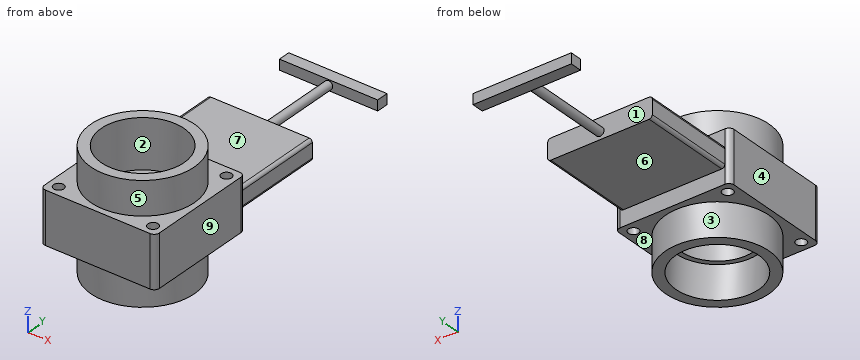
```python
from build123d import *

# Parameters (mm, degrees)
F0_R           = 50.00625
F0_R_2         = 40
F1_DEPTH       = 114.3
F3_R           = 50.00625
F4_DEPTH       = 25
F4_DEPTH_BACK  = 25
F5_R           = 5
F6_DEPTH       = 82.151
F8_DEPTH       = 90
F9_R           = 4
F10_DEPTH      = 85
F11_W          = 95
F11_H          = 10
F11_R          = 4
F12_DEPTH      = 11.51
F13_R          = 40
F13_R_2        = 35
F14_DEPTH      = 10
F14_DEPTH_BACK = 25


with BuildPart() as f1:
    # F0 (on Top) → F1 (new body)
    with BuildSketch(Plane.XY):
        Circle(F0_R)
        Circle(F0_R_2, mode=Mode.SUBTRACT)
    extrude(amount=F1_DEPTH)

    # F3 (on offset) → F4 (join, two sides)
    with BuildSketch(Plane.XY.offset(57.15)) as f4_sk:
        with BuildLine():
            ThreePointArc((55.5625, 50.5625), (54.0980339059, 54.0980339059), (50.5625, 55.5625))
            Line((50.5625, 55.5625), (-50.5625, 55.5625))
            ThreePointArc((-50.5625, 55.5625), (-54.0980339059, 54.0980339059), (-55.5625, 50.5625))
            Line((-55.5625, 50.5625), (-55.5625, -50.5625))
            ThreePointArc((-55.5625, -50.5625), (-54.0980339059, -54.0980339059), (-50.5625, -55.5625))
            Line((-50.5625, -55.5625), (50.5625, -55.5625))
            ThreePointArc((50.5625, -55.5625), (54.0980339059, -54.0980339059), (55.5625, -50.5625))
            Line((55.5625, -50.5625), (55.5625, 50.5625))
        make_face()
        Circle(F3_R, mode=Mode.SUBTRACT)
    extrude(amount=F4_DEPTH)
    extrude(f4_sk.sketch, amount=-F4_DEPTH_BACK)

    # F5 (on face) → F6 (cut, through all)
    with BuildSketch(Plane.XY.offset(82.15)):
        with Locations((-45.5625, 45.5625)):
            Circle(F5_R)
        with Locations((-45.5625, -45.5625)):
            Circle(F5_R)
        with Locations((45.5625, -45.5625)):
            Circle(F5_R)
        with Locations((45.5625, 45.5625)):
            Circle(F5_R)
    extrude(amount=-F6_DEPTH, mode=Mode.SUBTRACT)

    # F7 (on face) → F8 (join)
    with BuildSketch(Plane(origin=(0, 55.5625, 0), x_dir=(-1, 0, 0), z_dir=(0, 1, 0))):
        with BuildLine():
            Line((-47.5625, 47.15), (47.5625, 47.15))
            ThreePointArc((47.5625, 47.15), (49.6838203436, 48.0286796564), (50.5625, 50.15))
            Line((50.5625, 50.15), (50.5625, 64.15))
            ThreePointArc((50.5625, 64.15), (49.6838203436, 66.2713203436), (47.5625, 67.15))
            Line((47.5625, 67.15), (-47.5625, 67.15))
            ThreePointArc((-47.5625, 67.15), (-49.6838203436, 66.2713203436), (-50.5625, 64.15))
            Line((-50.5625, 64.15), (-50.5625, 50.15))
            ThreePointArc((-50.5625, 50.15), (-49.6838203436, 48.0286796564), (-47.5625, 47.15))
        make_face()
    extrude(amount=F8_DEPTH)

    # F9 (on face) → F10 (join)
    with BuildSketch(Plane(origin=(0, 145.5625, 0), x_dir=(-1, 0, 0), z_dir=(0, 1, 0))):
        with Locations((0, 54.15)):
            Circle(F9_R)
    extrude(amount=F10_DEPTH)

    # F11 (on face) → F12 (join)
    with BuildSketch(Plane(origin=(0, 230.5625, 0), x_dir=(-1, 0, 0), z_dir=(0, 1, 0))):
        with Locations((0, 54.15)):
            Rectangle(F11_W, F11_H)
        with Locations((0, 54.15)):
            Circle(F11_R, mode=Mode.SUBTRACT)
        with Locations((0, 54.15)):
            Circle(F11_R)
    extrude(amount=F12_DEPTH)

    # F13 (on offset) → F14 (join, two sides)
    with BuildSketch(Plane.XY.offset(57.15)) as f14_sk:
        Circle(F13_R)
        Circle(F13_R_2, mode=Mode.SUBTRACT)
    extrude(amount=F14_DEPTH)
    extrude(f14_sk.sketch, amount=-F14_DEPTH_BACK)


solid = f1.part
```
Design review of the part built by this model. Coordinates are the model's own, in mm. Face numbers are marked on the shaded views. A direction names the side the tool comes from. Coordinates: 2 decimals unless noted, no trailing zeros. Write each loop counter-clockwise with the first axis right and the second up, starting at its lowest first coordinate (ties: lowest second). Pieces come first, ordered by that corner, then holes. Notation, with made-up numbers: M 36,-40 L 40,-40 A23 ccw 40,-28 Z; hole C 51.5,-23 d3. An arc over 180 degrees is marked long. Answer as a JSON object with one key per item and string values.
Item 1: Add section C-C, the plane y = 91. Give the boundary of the cut face in (x, z).
Outcome:
{"outline": "M -50.56,50.15 A3 ccw -47.56,47.15 L 47.56,47.15 A3 ccw 50.56,50.15 L 50.56,64.15 A3 ccw 47.56,67.15 L -47.56,67.15 A3 ccw -50.56,64.15 Z"}
Item 2: Add section B-B, the plane x = -15.5. State how many separate pieces and enclosed holes the cut face has, and give its area (3 significant figures).
Outcome:
{"separate pieces": "3", "enclosed holes": "0", "area": "5,540 mm²"}
Item 3: Insertion check: pin 1 Ø5 at (y, z) = (238, 56) entering from +X; pin 2 Ø13 at (x, y) = (45.56, -45.56) entering from +Z; pin 3 Ø15.5 at (y, z) = (120.5, 56.5) entering from -X. Each pin has a flat end and moves straight along its axis. Give the tip position at first contact, or say it passes through.
Outcome:
{"pin 1": "x = 47.5", "pin 2": "z = 82.15", "pin 3": "x = -50.56"}
Item 4: Add section D-D, the plane z = 70.5. Give the boundary of the cut face in (x, y).
Outcome:
{"outline": "M -55.56,-50.56 A5 ccw -50.56,-55.56 L 50.56,-55.56 A5 ccw 55.56,-50.56 L 55.56,50.56 A5 ccw 50.56,55.56 L -50.56,55.56 A5 ccw -55.56,50.56 Z; hole C -45.56,-45.56 d10; hole C -45.56,45.56 d10; hole C 0,0 d80; hole C 45.56,-45.56 d10; hole C 45.56,45.56 d10"}
Item 5: Draft analysis for pull direction X (two halves, no side actions). For the marked faces 1, 2, 3 and 4, state which applies: pulls with the +X half, pulls with the -X half, needs draft (parallel to the pull), parting line crosses it, or undercut.
Outcome:
{"face 1": "needs draft", "face 2": "undercut", "face 3": "parting line crosses it", "face 4": "pulls with the -X half"}
Item 6: Wall thickness on probe 1 along Y at (x, z) = (45, 66); probe 2 along Y at (x, z) = (0, 60); probe 3 along Y at (x, z) = (6, 52): over which ranges is each line inside the solid? List them lowest first.
Outcome:
{"probe 1": "-55.56 to -50.53, -40.59 to 40.59, 50.53 to 145.56", "probe 2": "-55.56 to -35, 35 to 145.56", "probe 3": "-55.56 to -34.48, 34.48 to 145.56, 230.56 to 242.07"}
Item 7: Add section A-A, the plane y = 0. Give the boundary of the cut face in (x, z).
Outcome:
{"outline": "M -55.56,32.15 L -50.01,32.15 L -50.01,0 L -40,0 L -40,32.15 L -35,32.15 L -35,67.15 L -40,67.15 L -40,114.3 L -50.01,114.3 L -50.01,82.15 L -55.56,82.15 Z; M 35,32.15 L 40,32.15 L 40,0 L 50.01,0 L 50.01,32.15 L 55.56,32.15 L 55.56,82.15 L 50.01,82.15 L 50.01,114.3 L 40,114.3 L 40,67.15 L 35,67.15 Z"}
Item 8: Machinability: for the marked faces 5, 6, 7, 8 and 9, which of the approach directions +Z, -Z, +X, -X, +Y, -Y give a long, thin tool a straight path to every point of the face, cutting with its end or side? Answer none if there is none.
Outcome:
{"face 5": "+Z", "face 6": "-Z, +X, -X, +Y", "face 7": "+Z, +X, -X, +Y", "face 8": "-Z", "face 9": "+Z, -Z, +X, +Y, -Y"}
